```python
from build123d import *

# Parameters (mm, degrees)
SKETCH1_R           = 8
BOSS_EXTRUDE1_DEPTH = 19
SKETCH2_R           = 2
CUT_EXTRUDE1_DEPTH  = 24
CHAMFER1_SIZE       = 1


with BuildPart() as part:
    # Sketch1 → Boss-Extrude1 (new body)
    with BuildSketch(Plane.XY):
        Circle(SKETCH1_R)
    extrude(amount=BOSS_EXTRUDE1_DEPTH)

    # Sketch2 → Cut-Extrude1 (cut, symmetric)
    with BuildSketch(Plane(origin=(0, 0, 0), x_dir=(1, 0, 0), z_dir=(0, 1, 0))):
        with Locations(Location((0, -12.221312154, 0), (0, 0, 270))):
            Circle(SKETCH2_R)
    extrude(amount=CUT_EXTRUDE1_DEPTH, both=True, mode=Mode.SUBTRACT)

    # Chamfer1
    chamfer1_edges = [part.edges().sort_by_distance(p)[0] for p in [
        (-8, 0, 19),
    ]]
    chamfer(chamfer1_edges, length=CHAMFER1_SIZE)


solid = part.part
```
CAD build for the part. Positions are in the model's coordinates, mm. Round coordinates to 2 decimals unless told otherwise and drop trailing zeros. Loops run counter-clockwise (first coordinate to the right, second up) from the corner with the lowest first, then second, coordinate; pieces in that order, holes last. Notation, with made-up numbers: M 74.25,1.25 L 95.25,1.25 A11 cw 95.25,6.25 Z; hole C 46,61.5 d5. An arc over 180 degrees is marked long. Return JSON: item names as keys, results as strings. Group by question number.
(1) Drop flat-ended pins along their axis: P1, Ø2, axis at x = 4, z = 4, coming from the +Y side; P2, Ø1, axis at y = 3, z = 9, coming from the -X side. Give the stop position or say it passes through.
(2) Wall check: probe 1 along Z at (x, y) = (0, -0.5); probe 2 along Z at (x, y) = (-1, 1); probe 3 along X at (y, z) = (5.5, 10.75). Give the ranges that are in metal, low to high. Write a range as [from, to].
(3) Mould opens along Z. For faces 1 (the flat face through (0, 0, 0)), 2 (the flat face through (0, 0, 19)), 3 (the cylindrical face through (-0.766, 0.112, 14.069)) say: +Z half, -Z half, draft (parallel to the pull), parting line (faces both ways), or undercut.
(4) Saw through at A-A, the plane x = 0. List the corners of the cut face in (y, z), and give its area (3 significant figures).
(5) Saw through at C-C, the plane z = 15.75. List the corners of the cut face in (x, y).
(6) Saw through at B-B, the plane y = 0. List the corners of the cut face in (x, z), and give its area (3 significant figures).
Answer list:
{
 "1": {"P1": "y = 7.42", "P2": "x = -7.6"},
 "2": {"probe 1": "[0, 10.22], [14.22, 19]", "probe 2": "[0, 10.49], [13.95, 19]", "probe 3": "[-5.81, -1.35], [1.35, 5.81]"},
 "3": {"face 1": "-Z half", "face 2": "+Z half", "face 3": "undercut"},
 "4": {"outline": "M -8,0 L 8,0 L 8,10.22 L -8,10.22 Z; M -8,14.22 L 8,14.22 L 8,18 L 7,19 L -7,19 L -8,18 Z", "area": "239 mm2"},
 "5": {"outline": "C 0,0 d16"},
 "6": {"outline": "M -8,0 L 8,0 L 8,18 L 7,19 L -7,19 L -8,18 Z; hole C 0,12.22 d4", "area": "290 mm2"}
}
